Here's how the part is built. I have some questions about the finished solid (model axes, mm). A direction names the side the tool comes from. Coordinates: 2 decimals unless noted, no trailing zeros. Write each loop counter-clockwise with the first axis right and the second up, starting at its lowest first coordinate (ties: lowest second). Pieces come first, ordered by that corner, then holes. Notation, with made-up numbers: M -8.5,69 L 4.5,69 A27 cw 4.5,91 Z; hole C 55.5,-21 d4. An arc over 180 degrees is marked long. Use a Markdown table: item, result.
```python
from build123d import *

# Parameters (mm, degrees)
SKETCH_R        = 12.5
PAD_DEPTH       = 8
SKETCH001_R     = 9.95
PAD001_DEPTH    = 18
SKETCH002_R     = 3.25
POCKET_DEPTH    = 26.001
SKETCH003_W     = 6.7
SKETCH003_H     = 6.7
POCKET001_DEPTH = 9
SKETCH004_R     = 8
POCKET002_DEPTH = 2
CHAMFER_SIZE    = 1
CHAMFER001_SIZE = 1


with BuildPart() as part:
    # Sketch → Pad (new body)
    with BuildSketch(Plane.XY):
        Circle(SKETCH_R)
    extrude(amount=PAD_DEPTH)

    # Sketch001 (on Face3 of Pad) → Pad001 (join)
    with BuildSketch(Plane.XY.offset(8)):
        Circle(SKETCH001_R)
    extrude(amount=PAD001_DEPTH)

    # Sketch002 (on Face2 of Pad001) → Pocket (cut, through all)
    with BuildSketch(Plane(origin=(0, 0, 0), x_dir=(1, 0, 0), z_dir=(0, 0, -1))):
        Circle(SKETCH002_R)
        with BuildLine():
            Line((10, 7.5), (10, -7.5))
            ThreePointArc((10, -7.5), (12.5, 0), (10, 7.5))
        make_face()
    extrude(amount=-POCKET_DEPTH, mode=Mode.SUBTRACT)

    # Sketch003 (on Face2 of Pocket) → Pocket001 (cut)
    with BuildSketch(Plane(origin=(0, 0, 0), x_dir=(1, 0, 0), z_dir=(0, 0, -1))):
        Rectangle(SKETCH003_W, SKETCH003_H)
    extrude(amount=-POCKET001_DEPTH, mode=Mode.SUBTRACT)

    # Sketch004 → Pocket002 (cut)
    with BuildSketch(Plane(origin=(0, 0, 0), x_dir=(1, 0, 0), z_dir=(0, 0, -1))):
        Circle(SKETCH004_R)
    extrude(amount=-POCKET002_DEPTH, mode=Mode.SUBTRACT)

    # Chamfer
    chamfer_edges = [part.edges().sort_by_distance(p)[0] for p in [
        (-12.5, 0, 0),
        (10, 0, 0),
    ]]
    chamfer(chamfer_edges, length=CHAMFER_SIZE)

    # Chamfer001
    chamfer001_edges = [part.edges().sort_by_distance(p)[0] for p in [
        (-9.95, 0, 26),
    ]]
    chamfer(chamfer001_edges, length=CHAMFER001_SIZE)


solid = part.part
```
1. Will these pins go through, and if not, where does the flat tip stop? pin 1 Ø5 at (y, z) = (-5.5, 22) entering from -X; pin 2 Ø12 at (y, z) = (4.5, 20.5) entering from +X; pin 3 Ø12 at (x, z) = (-8.5, 16) entering from +Y; pin 4 Ø8 at (x, y) = (4, -1.5) entering from -Z.
Answers follow:
| item | result |
|---|---|
| pin 1 | stops at x = -9.49 |
| pin 2 | stops at x = 9.95 |
| pin 3 | stops at y = 9.63 |
| pin 4 | stops at z = 0 |
2. Suppose I cut it at A-A on y = 0. Write out the boundary of the cut face in (x, z).
Answers follow:
| item | result |
|---|---|
| outline | M -12.5,1 L -11.5,0 L -8,0 L -8,2 L -3.35,2 L -3.35,9 L -3.25,9 L -3.25,26 L -8.95,26 L -9.95,25 L -9.95,8 L -12.5,8 Z; M 3.25,9 L 3.35,9 L 3.35,2 L 8,2 L 8,0 L 9,0 L 10,1 L 10,8 L 9.95,8 L 9.95,25 L 8.95,26 L 3.25,26 Z |
3. Which directions (+Z, -Z, +X, -X, +Y, -Y) give clear straight access to the entire face, cutting with the end or side of a thin tool? Please do faces 1 (the face through (-10, -3, 8)), 2 (the face through (9.5, -0.1, 0.5)), 3 (the face through (-3.35, 0, 5)).
Answers follow:
| item | result |
|---|---|
| face 1 | +Z |
| face 2 | -Z, +X, +Y, -Y |
| face 3 | -Z |
4. Suppose I cut it at C-C on z = 13. Write out the boundary of the cut face in (x, y), and give its area (3 significant figures).
Answers follow:
| item | result |
|---|---|
| outline | C 0,0 d19.9; hole C 0,0 d6.5 |
| area | 278 mm2 |
5. We'd pull the mould along Y, two halves only. Please class faces 4 (the face through (0, -3.35, 5)), 5 (the face through (-7.9, -6.05, 16.38)), 6 (the face through (4, 0, 26)): +Y half, -Y half, draft (parallel to the pull), parting line (faces both ways), or undercut.
Answers follow:
| item | result |
|---|---|
| face 4 | undercut |
| face 5 | parting line |
| face 6 | draft |
6. I need wall thicknesses on probe 1 along Y at (x, z) = (0, 1.35); probe 2 along X at (y, z) = (0, 1); probe 3 along Y at (x, z) = (0, 18.25). Which ranges of each line are inside material? Lowest first, please.
Answers follow:
| item | result |
|---|---|
| probe 1 | y = -12.5 to -8, 8 to 12.5 |
| probe 2 | x = -12.5 to -8, 8 to 10 |
| probe 3 | y = -9.95 to -3.25, 3.25 to 9.95 |
7. Suppose I cut it at B-B on x = 0. Write out the boundary of the cut face in (y, z).
Answers follow:
| item | result |
|---|---|
| outline | M -12.5,1 L -11.5,0 L -8,0 L -8,2 L -3.35,2 L -3.35,9 L -3.25,9 L -3.25,26 L -8.95,26 L -9.95,25 L -9.95,8 L -12.5,8 Z; M 3.25,9 L 3.35,9 L 3.35,2 L 8,2 L 8,0 L 11.5,0 L 12.5,1 L 12.5,8 L 9.95,8 L 9.95,25 L 8.95,26 L 3.25,26 Z |
